Autodesk Inventor part; units mm, degrees
ref_plane "YZ Plane" through (0, 0, 0) normal (1, 0, 0) x (0, 1, 0)
ref_plane "XZ Plane" through (0, 0, 0) normal (0, 1, 0) x (-1, 0, 0)
ref_plane "XY Plane" through (0, 0, 0) normal (0, 0, 1) x (1, 0, 0)
sketch "Sketch1" plane through (0, 0, 0) normal (1, 0, 0) x (0, 1, 0)
  line L0 (0, 0) -> (8.5858, 0)
  line L1 (8.5858, 0) -> (10, 1.4142)
  line L2 (10, 1.4142) -> (10, 3.4142)
  line L3 (10, 3.4142) -> (8, 3.4142)
  line L4 (8, 3.4142) -> (8, 20)
  line L5 (8, 20) -> (0, 20)
  line L6 (0, 20) -> (0, 0)
  dimension "d1" = 16
  dimension "d2" = 2
  dimension "d3" = 2
  dimension "d4" = 45
  dimension "d5" = 20
revolve "Revolution1" add sketch "Sketch1" angle 360 about axis through (0, 0, 20) along (0, 0, -1)
sketch "Sketch2" plane through (0, 0, 0) normal (0, 0, -1) x (-1, 0, 0)
  circle A0 centre (0, 0) radius 8.5858
  circle A1 centre (0, 0) radius 8.0858
  circle A2 centre (0, 0) radius 7.0858
  dimension "d7" = 0.5
  dimension "d8" = 1
extrude "Extrusion1" cut sketch "Sketch2" against normal blind 0.1 contours A1
properties part number "Power Button" material "Stainless Steel"
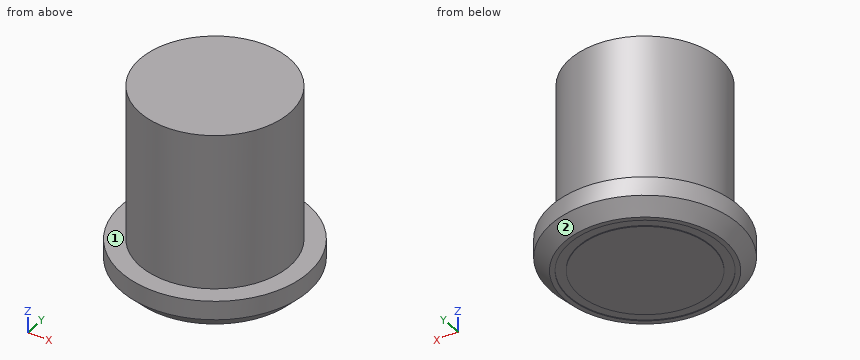
Input: part model. Units: mm. Frame: model coordinates. Face numbers are marked on the shaded views. A direction names the side the tool comes from. Coordinates: 2 decimals unless noted, no trailing zeros. Order: outer loops, then holes, each group sorted by start corner. A loop starts at its lowest first (then second) coordinate and runs counter-clockwise, first axis right, second up.
1. Cut plane C-C, the plane z = 2. Return loops of the section in (x, y), plus the area to 3 significant figures.
Checked values:
outline: circle Ø20 at (0, 0)
area: 314 mm2
2. Cut plane B-B, the plane z = 16. Return loops of the section in (x, y).
Checked values:
outline: circle Ø16 at (0, 0)
3. Ray query, line 1 along Y through (x, z) = (0, 0.05); line 2 along Z through (x, y) = (7.75, 3.25); line 3 along Z through (x, y) = (5.75, -4.5). Return the intervals inside material, ascending.
Checked values:
line 1: y = -8.64 to -8.09, -7.09 to 7.09, 8.09 to 8.64
line 2: z = 0 to 3.41
line 3: z = 0.1 to 20
4. Cut plane A-A, the plane x = 0. Return loops of the section in (y, z).
Checked values:
outline: (-10, 1.41) - (-8.59, 0) - (-8.09, 0) - (-8.09, 0.1) - (-7.09, 0.1) - (-7.09, 0) - (7.09, 0) - (7.09, 0.1) - (8.09, 0.1) - (8.09, 0) - (8.59, 0) - (10, 1.41) - (10, 3.41) - (8, 3.41) - (8, 20) - (-8, 20) - (-8, 3.41) - (-10, 3.41) - close
5. Contact query for flat-ended pins moving along their axis: P1, Ø3, axis at x = -2.5, z = 5.5, coming from the -Y side; P2, Ø10, axis at y = 7, z = 4.5, coming from the -X side; P3, Ø6, axis at y = -4, z = 15, coming from the -X side. Output: stop coordinate, or through.
Checked values:
P1: stops at y = -7.94
P2: stops at x = -9.77
P3: stops at x = -7.94
6. Access query for the marked faces 1 and 2. Directions: +Z, -Z, +X, -X, +Y, -Y. A direction counts if a zero-diameter tool reaches every point of the face in a straight line with its end or side. Return the directions, or none.
Checked values:
face 1: +Z
face 2: -Z
